```python
from build123d import *

# Parameters (mm, degrees)
RESSALTO_EXTRUS_O1_DEPTH = 100
ESBO_O2_R                = 1.75
CORTE_EXTRUS_O1_DEPTH    = 100
PADR_O_LINEAR1_COUNT     = 8
PADR_O_LINEAR1_PITCH     = 12.714285714
ESBO_O3_R                = 1.75
CORTE_EXTRUS_O2_DEPTH    = 100
PADR_O_LINEAR2_COUNT     = 8
PADR_O_LINEAR2_PITCH     = 12.714285714
CHANFRO1_SIZE            = 2


with BuildPart() as part:
    # Esboço1 → Ressalto-extrusão1 (new body)
    with BuildSketch(Plane.XY):
        Polygon((0, 0), (0, 15), (4, 15), (4, 4), (15, 4), (15, 0), align=None)
    extrude(amount=RESSALTO_EXTRUS_O1_DEPTH)

    # Esboço2 → Corte-extrusão1 (cut)
    with BuildSketch(Plane(origin=(4, 0, 0), x_dir=(0, 0, -1), z_dir=(1, 0, 0))):
        with Locations((-94.5, 9.5)):
            Circle(ESBO_O2_R)
    corte_extrus_o1 = extrude(amount=-CORTE_EXTRUS_O1_DEPTH, mode=Mode.SUBTRACT)

    # Padrão linear1: Corte-extrusão1 ×8
    with Locations(*[(0, 0, -i * PADR_O_LINEAR1_PITCH) for i in range(1, PADR_O_LINEAR1_COUNT)]):
        add(corte_extrus_o1, mode=Mode.SUBTRACT)

    # Esboço3 → Corte-extrusão2 (cut)
    with BuildSketch(Plane(origin=(0, 4, 0), x_dir=(1, 0, 0), z_dir=(0, 1, 0))):
        with Locations((9.5, -94.5)):
            Circle(ESBO_O3_R)
    corte_extrus_o2 = extrude(amount=-CORTE_EXTRUS_O2_DEPTH, mode=Mode.SUBTRACT)

    # Padrão linear2: Corte-extrusão2 ×8
    with Locations(*[(0, 0, -i * PADR_O_LINEAR2_PITCH) for i in range(1, PADR_O_LINEAR2_COUNT)]):
        add(corte_extrus_o2, mode=Mode.SUBTRACT)

    # Chanfro1
    chanfro1_edges = [part.edges().sort_by_distance(p)[0] for p in [
        (4, 4, 50),
    ]]
    chamfer(chanfro1_edges, length=CHANFRO1_SIZE)


solid = part.part
```
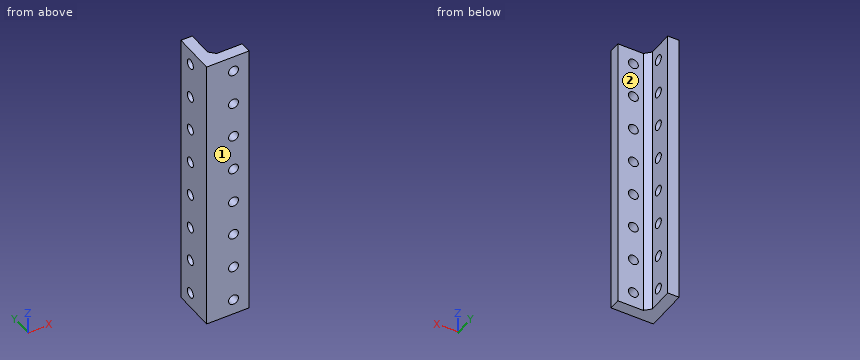
Design review of the part built by this model. Coordinates are the model's own, in mm. Face numbers are marked on the shaded views. A direction names the side the tool comes from. Give positions to 0.01 mm unless a question says otherwise; leave off trailing zeros. Order: outer loops, then holes, each group sorted by start corner. A loop starts at its lowest first (then second) coordinate and runs counter-clockwise, first axis right, second up. Notation, with made-up numbers: M 0.25,19.25 L 59.25,19.25 A11 cw 59.25,28.25 Z; hole C 14,37.5 d8. An arc over 180 degrees is marked long. One line per question, with ' | ' between items. Start each with the question number.
Q1. For L1, parallel to Y at x = 1.75, z = 5.5; L2, parallel to X at y = 10.75, z = 7, list the stretches that pass through material, from the lowest coordinate up. Write a range as [from, to].
Q2. Machinability: for the marked faces 1 and 2, which of the approach directions +Z, -Z, +X, -X, +Y, -Y give a long, thin tool a straight path to every point of the face, cutting with its end or side? Answer none if there is none.
Q3. We need section C-C (x = 9.5). State how many separate pieces and enclosed holes the cut face has, plus the area to 3 significant figures.
Q4. We need section B-B (z = 79). Write out the cut boundary in (x, y), plus the area to 3 significant figures.
Q5. We need section A-A (z = 94.5). Write out the cut boundary in (x, y), plus the area to 3 significant figures.
Q6. For pin 1 Ø5.5 at (x, z) = (9.5, 81.79) entering from +Y; pin 2 Ø4.5 at (y, z) = (9.5, 30.93) entering from +X, all flat-tipped, find the tip position at first contact; note any pin that passes through.
Returned:
1) L1: [0, 7.75], [11.25, 15] | L2: [0, 4]
2) face 1: +Z, -Z, +X, -X, -Y | face 2: +Z, -Z, +X, +Y
3) separate pieces: 9 | enclosed holes: 0 | area: 288 mm2
4) outline: M 0,0 L 15,0 L 15,4 L 6,4 L 4,6 L 4,15 L 0,15 Z | area: 106 mm2
5) outline: M 0,0 L 7.75,0 L 7.75,4 L 6,4 L 4,6 L 4,7.75 L 0,7.75 Z; M 0,11.25 L 4,11.25 L 4,15 L 0,15 Z; M 11.25,0 L 15,0 L 15,4 L 11.25,4 Z | area: 78.0 mm2
6) pin 1: y = 4 | pin 2: x = 4
